Verification items for the finished model (mm, model axes). A direction names the side the tool comes from. Give positions to 0.01 mm unless a question says otherwise; leave off trailing zeros. Write each loop counter-clockwise with the first axis right and the second up, starting at its lowest first coordinate (ties: lowest second). Pieces come first, ordered by that corner, then holes. Notation, with made-up numbers: (35, 78.5) - (85, 78.5) arc R35 cw to (85, 113.5) - close; hole circle Ø7 at (3.5, 74). An arc over 180 degrees is marked (long way). Answer as a JSON object with one key per item and string values. Group by question number.
Item 1: Tool access check on faces 1 (the face through (6, 40, 20)), 2 (the face through (6.08, 67.15, 16.99)), 3 (the face through (6.08, 13.01, -22.85)), 4 (the face through (8, 100, 0)). Record the directions out of +Z, -Z, +X, -X, +Y, -Y that give a thin tool (end or side, any length) a straight path to the whole face; none if there is none.
Item 2: Scan lines: line 1 along Y through (x, z) = (11, 45); line 2 along X through (y, z) = (57, 0.5); line 3 along Y through (x, z) = (7, 40). Record each from-to range of solid material in increasing order. Write a range as [from, to].
Item 3: Sectioned sample at A-A, the plane z = -15. Record the boundary of the cut face in (x, y).
Item 4: Sectioned sample at D-D, the plane z = -50. Record the boundary of the cut face in (x, y).
Item 5: Go/stop test with flat-tipped pins: pin 1 (1.6 mm diameter, centred on x = 10, z = 50, fed in from +Y); pin 2 (3 mm diameter, centred on x = 2.5, y = 77.5, fed in from -Z); pin 3 (6 mm diameter, centred on x = 6.5, y = 44, fed in from +Z). Record where each tip stops, or that it passes through.
Item 6: Sectioned sample at C-C, the plane z = 0. Record the boundary of the cut face in (x, y).
Item 7: Draft check along Y on faces 5 (the face through (6.08, 89.1, -19.14)), 6 (the face through (6, -10, 1)), 7 (the face through (10, 40, 0)), 8 (the face through (12, 0, -61)). Enter one of: +Y half, -Y half, draft (parallel to the pull), parting line (faces both ways), or undercut.
Autodesk Inventor part; units mm, degrees
ref_plane "YZ Plane" through (0, 0, 0) normal (1, 0, 0) x (0, 1, 0)
ref_plane "XZ Plane" through (0, 0, 0) normal (0, 1, 0) x (-1, 0, 0)
ref_plane "XY Plane" through (0, 0, 0) normal (0, 0, 1) x (1, 0, 0)
sketch "Sketch1" plane through (0, 0, 0) normal (1, 0, 0) x (0, 1, 0)
  line L0 (-10, -70) -> (10, -70)
  line L1 (10, -70) -> (10, 70)
  line L2 (10, 70) -> (-10, 70)
  line L3 (-10, 70) -> (-10, -70)
  line L4 (-10, -70) -> (10, 70) construction
  line L5 (10, -70) -> (-10, 70) construction
  line L6 (10, 0) -> (70, 0)
  line L7 (70, 0) -> (70, 20)
  line L8 (70, 20) -> (10, 20)
  line L9 (10, 20) -> (10, 0)
  line L10 (70, 0) -> (70, -20)
  line L11 (70, -20) -> (10, -20)
  line L12 (10, -20) -> (10, 0)
  line L13 (90, 20) -> (110, 20)
  line L14 (110, 20) -> (110, -20)
  line L15 (110, -20) -> (90, -20)
  line L16 (90, -20) -> (90, 20)
  line L17 (110, -20) -> (50, -20)
  line L18 (50, -20) -> (50, -40)
  line L19 (50, -40) -> (110, -40)
  line L20 (110, -40) -> (110, -20)
  point P0 (0, 0)
  point P1 (90, -20)
  point P2 (70, -20)
  point P3 (50, -20)
  dimension "d0" = 20
  dimension "d1" = 140
  dimension "d2" = 80
  dimension "d3" = 20
  dimension "d17" = 60
  dimension "d18" = 20
  dimension "d19" = 20
  dimension "d20" = 20
extrude "Extrusion1" add sketch "Sketch1" along normal blind 12
fillet "Fillet1" radius 10 10 edges at (6, 10, 70) (6, 10, -70) (6, 10, 20) (6, 10, -20) (6, 70, 20) (6, 90, 20) (6, 110, 20) (6, 110, -40) (6, 50, -40) (6, 50, -20)
fillet "Fillet1" radius 3 2 edges at (6, 70, -20) (6, 90, -20)
sketch "Sketch2" plane through (0, 10, 60) normal (0, 1, 0) x (1, 0, 0)
  line L0 (12, -10) -> (12, 130)
  line L1 (0, -10) -> (12, -10)
  line L2 (12, 130) -> (0, 130)
  point P0 (0, 60)
  point P1 (12, 10)
  point P2 (12, 110)
  dimension "d7" = 100
  dimension "d8" = 20
  dimension "d9" = 20
hole "Hole1" at (12, 10, 50) at (12, 10, -50) direction (0, -1, 0) diameter 5 end through all counterbore diameter 11 counterbore depth 2
sketch "Sketch3" plane through (0, 110, 10) normal (0, 1, 0) x (1, 0, 0)
  line L0 (12, -37.5) -> (12, 57.5)
  point P0 (0, 10)
  point P1 (12, 10)
hole "Hole2" at (12, 110, 0) direction (0, -1, 0) diameter 8 depth 70
sketch "Sketch4" plane through (0, -10, -70) normal (0, -1, 0) x (1, 0, 0)
  arc A0 (12, 122.5) -> (12, 117.5) centre (12, 120) ccw
  arc A1 (12, 22.5) -> (12, 17.5) centre (12, 20) ccw
  point P0 (0, 70)
hole "Hole3" at (12, -10, 50) at (12, -10, -50) direction (0, 1, 0) diameter 11 depth 2
properties part number "clamp"
Geometry check:
{
 "1": {"face 1": "+Z, +X, -X, +Y", "face 2": "+Z, +X, -X", "face 3": "-Z, +X, -X", "face 4": "+X, +Y"},
 "2": {"line 1": "[-8, 8]", "line 2": "[0, 8.03]", "line 3": "[-10, 10]"},
 "3": {"outline": "(0, -10) - (12, -10) - (12, 70) - (0, 70) - close; (0, 90) - (12, 90) - (12, 110) - (0, 110) - close"},
 "4": {"outline": "(0, -10) - (6.5, -10) - (6.5, -8) - (9.5, -8) - (9.5, 8) - (6.5, 8) - (6.5, 10) - (0, 10) - close"},
 "5": {"pin 1": "y = 8", "pin 2": "z = -40", "pin 3": "z = 20"},
 "6": {"outline": "(0, -10) - (12, -10) - (12, 40) - (8, 40) - (8, 70) - (0, 70) - close; (0, 90) - (8, 90) - (8, 110) - (0, 110) - close"},
 "7": {"face 5": "undercut", "face 6": "-Y half", "face 7": "+Y half", "face 8": "draft"}
}
